Can you work these out from the model? Positions are in its coordinate system, mm. Give positions to 0.01 mm unless a question says otherwise; leave off trailing zeros. Loops run counter-clockwise (first coordinate to the right, second up) from the corner with the lowest first, then second, coordinate; pieces in that order, holes last.
from build123d import *

# Parameters (mm, degrees)
SKETCH1_W                  = 78
SKETCH1_H                  = 120
MAIN_SLIDER_BOTTOM_DEPTH   = 2
SLIDER_BOTTOM_CONTOURING_R = 4


with BuildPart() as part:
    # Sketch1 → Main Slider Bottom (new body)
    with BuildSketch(Plane.XY):
        with Locations((39, 60)):
            Rectangle(SKETCH1_W, SKETCH1_H)
        with BuildLine():
            Line((40.118033989, 4), (46, 4))
            Line((46, 4), (46, 2))
            Line((46, 2), (40.118033989, 2))
            ThreePointArc((40.118033989, 2), (39, 1.5), (37.881966011, 2))
            Line((37.881966011, 2), (32, 2))
            Line((32, 2), (32, 4))
            Line((32, 4), (37.881966011, 4))
            ThreePointArc((37.881966011, 4), (39, 4.5), (40.118033989, 4))
        make_face(mode=Mode.SUBTRACT)
        with BuildLine():
            Line((40.118033989, 118), (46, 118))
            Line((46, 118), (46, 116))
            Line((46, 116), (40.118033989, 116))
            ThreePointArc((40.118033989, 116), (39, 115.5), (37.881966011, 116))
            Line((37.881966011, 116), (32, 116))
            Line((32, 116), (32, 118))
            Line((32, 118), (37.881966011, 118))
            ThreePointArc((37.881966011, 118), (39, 118.5), (40.118033989, 118))
        make_face(mode=Mode.SUBTRACT)
        with BuildLine():
            Line((74, 97.118033989), (74, 103))
            Line((74, 103), (76, 103))
            Line((76, 103), (76, 97.118033989))
            ThreePointArc((76, 97.118033989), (76.5, 96), (76, 94.881966011))
            Line((76, 94.881966011), (76, 89))
            Line((76, 89), (74, 89))
            Line((74, 89), (74, 94.881966011))
            ThreePointArc((74, 94.881966011), (73.5, 96), (74, 97.118033989))
        make_face(mode=Mode.SUBTRACT)
        with BuildLine():
            Line((4, 97.118033989), (4, 103))
            Line((4, 103), (2, 103))
            Line((2, 103), (2, 97.118033989))
            ThreePointArc((2, 97.118033989), (1.5, 96), (2, 94.881966011))
            Line((2, 94.881966011), (2, 89))
            Line((2, 89), (4, 89))
            Line((4, 89), (4, 94.881966011))
            ThreePointArc((4, 94.881966011), (4.5, 96), (4, 97.118033989))
        make_face(mode=Mode.SUBTRACT)
        with BuildLine():
            Line((2, 22.881966011), (2, 17))
            Line((2, 17), (4, 17))
            Line((4, 17), (4, 22.881966011))
            ThreePointArc((4, 22.881966011), (4.5, 24), (4, 25.118033989))
            Line((4, 25.118033989), (4, 31))
            Line((4, 31), (2, 31))
            Line((2, 31), (2, 25.118033989))
            ThreePointArc((2, 25.118033989), (1.5, 24), (2, 22.881966011))
        make_face(mode=Mode.SUBTRACT)
        with BuildLine():
            Line((74, 22.881966011), (74, 17))
            Line((74, 17), (76, 17))
            Line((76, 17), (76, 22.881966011))
            ThreePointArc((76, 22.881966011), (76.5, 24), (76, 25.118033989))
            Line((76, 25.118033989), (76, 31))
            Line((76, 31), (74, 31))
            Line((74, 31), (74, 25.118033989))
            ThreePointArc((74, 25.118033989), (73.5, 24), (74, 22.881966011))
        make_face(mode=Mode.SUBTRACT)
    extrude(amount=MAIN_SLIDER_BOTTOM_DEPTH)

    # Slider Bottom Contouring
    slider_bottom_contouring_edges = [part.edges().sort_by_distance(p)[0] for p in [
        (0, 120, 1),
        (78, 120, 1),
        (78, 0, 1),
        (0, 0, 1),
    ]]
    fillet(slider_bottom_contouring_edges, radius=SLIDER_BOTTOM_CONTOURING_R)


solid = part.part
(1) Suppose I cut it at A-A on y = 99. List the corners of the cut face in (x, z) for me, plus the area to 3 significant figures.
Returned:
outline: (0, 0) - (2, 0) - (2, 2) - (0, 2) - close; (4, 0) - (74, 0) - (74, 2) - (4, 2) - close; (76, 0) - (78, 0) - (78, 2) - (76, 2) - close
area: 148 mm2
(2) Suppose I cut it at B-B on x = 34.5. List the corners of the cut face in (y, z) for me.
Returned:
outline: (0, 0) - (2, 0) - (2, 2) - (0, 2) - close; (4, 0) - (116, 0) - (116, 2) - (4, 2) - close; (118, 0) - (120, 0) - (120, 2) - (118, 2) - close
(3) Suppose I cut it at C-C on z = 1.4. Give the number of separate pieces and of enclosed holes in the cut face, plus the area to 3 significant figures.
Returned:
separate pieces: 1
enclosed holes: 6
area: 9,170 mm2
(4) Will these pins go through, and if not, where does the flat tip stop? P1, Ø0.6, axis at y = 3, z = 1, coming from the +X side; P2, Ø1, axis at x = 75.5, z = 0.5, coming from the +Y side.
Returned:
P1: stops at x = 77.94
P2: stops at y = 119.87
(5) Please list where these lines run through material, in increasing order: probe 1 along Y at (x, z) = (36, 1.4); probe 2 along Y at (x, z) = (38.5, 0.5).
Returned:
probe 1: y = 0 to 2, 4 to 116, 118 to 120
probe 2: y = 0 to 1.59, 4.41 to 115.59, 118.41 to 120
